```python
from build123d import *

# Parameters (mm, degrees)
SKETCH1_W                  = 76.2
SKETCH1_H                  = 76.2
BOSS_EXTRUDE1_DEPTH        = 12.7
F_10_32_TAPPED_HOLE1_D     = 4.0386
F_10_32_TAPPED_HOLE1_DEPTH = 9.652
F_10_32_TAPPED_HOLE1_TIP   = 1.213317848
F_10_32_TAPPED_HOLE2_D     = 4.0386
SKETCH9_R                  = 7.9375
CUT_EXTRUDE2_DEPTH         = 56.358016583
FILLET1_R                  = 38.1
SKETCH10_R                 = 3.175
CUT_EXTRUDE3_DEPTH         = 56.358016583


with BuildPart() as part:
    # Sketch1 → Boss-Extrude1 (new body)
    with BuildSketch(Plane(origin=(0, 0, 0), x_dir=(1, 0, 0), z_dir=(0, 1, 0))):
        Rectangle(SKETCH1_W, SKETCH1_H)
    extrude(amount=BOSS_EXTRUDE1_DEPTH)

    # #10-32 Tapped Hole1
    with Locations(Plane(origin=(38.1, 0, 0), x_dir=(0, 0, -1), z_dir=(1, 0, 0))):
        with Locations((-25.4, 6.35), (25.4, 6.35)):
            Hole(F_10_32_TAPPED_HOLE1_D / 2, depth=F_10_32_TAPPED_HOLE1_DEPTH)
            with Locations((0, 0, -(F_10_32_TAPPED_HOLE1_DEPTH + F_10_32_TAPPED_HOLE1_TIP / 2))):  # 118° drill point
                Cone(0, F_10_32_TAPPED_HOLE1_D / 2, F_10_32_TAPPED_HOLE1_TIP, mode=Mode.SUBTRACT)

    # #10-32 Tapped Hole2 (through all)
    with Locations(Plane(origin=(0, 12.7, 0), x_dir=(1, 0, 0), z_dir=(0, 1, 0))):
        with Locations((-23.5966, -23.5966), (-23.5966, 23.5966), (23.5966, 23.5966), (23.5966, -23.5966)):
            Hole(F_10_32_TAPPED_HOLE2_D / 2)

    # Sketch9 → Cut-Extrude2 (cut, through all)
    with BuildSketch(Plane(origin=(0, 12.7, 0), x_dir=(1, 0, 0), z_dir=(0, 1, 0))):
        with Locations(Location((0, 0, 0), (0, 0, 270))):
            Circle(SKETCH9_R)
    extrude(amount=-CUT_EXTRUDE2_DEPTH, mode=Mode.SUBTRACT)

    # Fillet1
    fillet1_edges = [part.edges().sort_by_distance(p)[0] for p in [
        (-38.1, 6.35, -38.1),
        (-38.1, 6.35, 38.1),
    ]]
    fillet(fillet1_edges, radius=FILLET1_R - 0.0001)  # a hair under: the kernel refuses the full size

    # Sketch10 → Cut-Extrude3 (cut, through all)
    with BuildSketch(Plane(origin=(0, 0, 0), x_dir=(0, 0, -1), z_dir=(1, 0, 0))):
        with Locations(Location((0, 6.35, 0), (0, 0, 180))):
            Circle(SKETCH10_R)
    extrude(amount=CUT_EXTRUDE3_DEPTH, mode=Mode.SUBTRACT)


solid = part.part
```
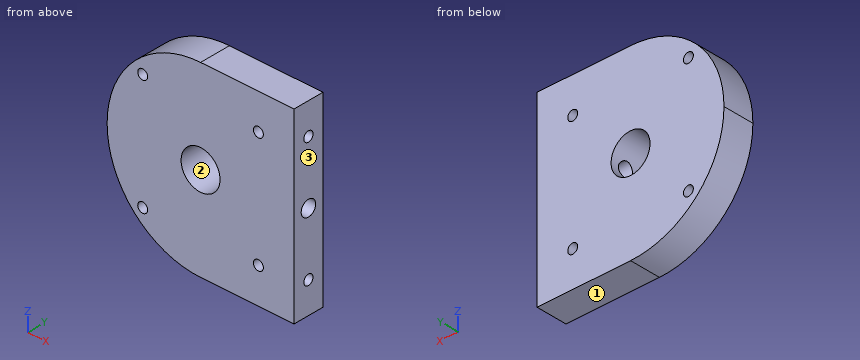
Design review of the part built by this model. Coordinates are the model's own, in mm. Face numbers are marked on the shaded views. Give positions to 0.01 mm unless a question says otherwise; leave off trailing zeros. Order: outer loops, then holes, each group sorted by start corner. A loop starts at its lowest first (then second) coordinate and runs counter-clockwise, first axis right, second up. Notation, with made-up numbers: (71.5, -34.5) -> (86.5, -34.5) arc R32 cw to (86.5, 4.5) -> close; hole circle Ø11 at (-30, -12). An arc over 180 degrees is marked (long way). Write each question's results on one line, items separated by ' | '. Start each with the question number.
Q1. Mouldability with a two-part tool opening along X and no side actions: class the marked faces 1, 2 and 3 as +X half, -X half, draft (parallel to the pull), parting line (faces both ways), or undercut.
Q2. Add section A-A on z = -5. Give the boundary of the cut face in (x, y).
Q3. Add section C-C on y = 2.25. State how many separate pieces and enclosed holes the cut face has, and give its area (3 significant figures).
Q4. Add section B-B on x = 12. Give the boundary of the cut face in (y, z) (3 decimals), and give its area (3 significant figures).
Q5. For pin 1 (3 mm diameter, centred on x = 23.6, z = 23.6, fed in from +Y); pin 2 (5.5 mm diameter, centred on y = 6.35, z = -25.4, fed in from -X); pin 3 (5 mm diameter, centred on y = 6.35, z = 0, fed in from +X); pin 4 (1 mm diameter, centred on y = 6.5, z = 6, fed in from -X), all flat-tipped, find the tip position at first contact; note any pin that passes through.
Q6. Wall thickness on L1, parallel to Z at x = 32.5, y = 6.35 (3 decimals); L2, parallel to Y at x = 19, z = 0 (3 decimals); L3, parallel to Z at x = 6.5, y = 3: over which ranges is each line inside the solid? List them lowest first. Write a range as from..to.
Found:
1) face 1: draft | face 2: undercut | face 3: +X half
2) outline: (-37.77, 0) -> (-6.16, 0) -> (-6.16, 12.7) -> (-37.77, 12.7) -> close; (6.16, 0) -> (38.1, 0) -> (38.1, 12.7) -> (6.16, 12.7) -> close
3) separate pieces: 1 | enclosed holes: 5 | area: 4,930 mm2
4) outline: (0, -38.1) -> (12.7, -38.1) -> (12.7, 38.1) -> (0, 38.1) -> close; hole circle Ø6.35 at (6.35, 0) | area: 936 mm2
5) pin 1: passes through | pin 2: stops at x = -30.64 | pin 3: stops at x = -7.53 | pin 4: stops at x = -37.7
6) L1: z = -38.1..-27.419, -23.381..-3.175, 3.175..23.381, 27.419..38.1 | L2: y = 0..3.175, 9.525..12.7 | L3: z = -38.1..-4.56, 4.56..38.1
